```python
from build123d import *

# Parameters (mm, degrees)
F0_W     = 37
F0_H     = 69
F1_DEPTH = 5


with BuildPart() as f1:
    # F0 (on Top) → F1 (new body)
    with BuildSketch(Plane.XY):
        Polygon((109.757393, -47.013952), (-190.469548, -47.013952), (-187.938355, -69.176264), (-184.088363, -77.644812), (-178.970914, -85.570573), (-173.10958, -92.22553), (-166.061834, -97.942505), (-158.033386, -102.625757), (-150.505585, -106.763709), (-142.395731, -109.967075), (-134.17314, -111.816847), (-125.182951, -113.624161), (-117.335529, -114.393513), (-110.297666, -113.927758), (-97.994511, -110.570822), (-84.98137, -104.478377), (-74.645462, -98.277857), (-61.347514, -92.467954), (-54.509754, -89.918709), (-46.818863, -88.209901), (-39.777415, -88.209901), (-33.070793, -88.209901), (-25.985741, -90.074082), (-18.618021, -92.997303), (-10.935776, -97.133205), (-1.40856, -104.7078), (7.10493, -112.998784), (15.743346, -121.422512), (21.768701, -126.512042), (30.47871, -133.017234), (39.396258, -138.681565), (50.354269, -144.791737), (60.591184, -149.491585), (74.199441, -154.41068), (89.423326, -158.059629), (98.85233, -159.107134), (106.677154, -159.976425), (116.486558, -159.976425), (126.872966, -159.103989), (140.423232, -157.318581), (153.42437, -154.017258), (167.162878, -148.336862), (175.342116, -143.532352), (185.6123, -136.302521), (195.518968, -128.048335), (204.653845, -117.358152), (213.371967, -105.595887), (220.455531, -93.514166), (225.775129, -81.625274), (230.597933, -67.78821), (233.441157, -55.785481), (235.624263, -44.975688), (236.896344, -20.704121), (236.86714, -9.510057), (236.86714, 1.11357), (235.906968, 22.984027), (233.25353, 44.31771), (229.252552, 63.059144), (223.510394, 79.554792), (216.840677, 92.894226), (207.739533, 107.33053), (197.024369, 120.1263), (184.641449, 131.468644), (171.094149, 140.879356), (153.60487, 149.05483), (132.97725, 154.472187), (114.898965, 156.457659), (99.067456, 156.457659), (84.663291, 154.488749), (66.679821, 149.783781), (53.734493, 144.398522), (42.264603, 138.037948), (27.751352, 128.291809), (16.359527, 119.536983), (4.246612, 108.496011), (-5.338126, 100.151649), (-13.215689, 95.496727), (-20.495536, 92.632523), (-29.407222, 90.433524), (-36.891697, 89.410468), (-42.068154, 89.410468), (-50.267792, 90.919179), (-59.070143, 93.618111), (-68.10425, 98.191586), (-78.777898, 104.228198), (-85.258181, 107.363312), (-92.926764, 110.724328), (-100.445934, 113.46735), (-107.684615, 114.975152), (-115.831575, 115.993351), (-123.636163, 115.993351), (-129.309204, 115.993351), (-133.603284, 114.941916), (-137.040821, 113.433007), (-138.448742, 112.306855), (-139.140668, 111.03855), (-139.344401, 110.549672), (-138.28696, 108.284083), (-136.043459, 105.957887), (-131.906646, 102.131959), (-126.94568, 97.960933), (-121.69705, 91.98096), (-117.6631, 84.796643), (-115.553754, 76.732782), (-114.52125, 64.899556), (-115.629325, 56.405594), (-116.508421, 53.80871), (109.757393, 52.986048), align=None)
        Polygon((241.896685, -20.828539), (241.86714, -9.503535), (241.86714, 1.223274), (240.893394, 23.402912), (238.188565, 45.149782), (234.077219, 64.408205), (228.126581, 81.502758), (221.202205, 95.35151), (211.789387, 110.282193), (200.645468, 123.589971), (187.770458, 135.383053), (173.597124, 145.228644), (155.312446, 153.775932), (133.890159, 159.40199), (115.172707, 161.457659), (98.727311, 161.457659), (83.688435, 159.40199), (65.079178, 154.533299), (51.555006, 148.90724), (39.653731, 142.307444), (24.831248, 132.353646), (13.146367, 123.3736), (0.920512, 112.229684), (-8.275919, 104.223377), (-15.416681, 100.003837), (-22.016478, 97.407195), (-30.347364, 95.35151), (-37.231842, 94.410468), (-41.61199, 94.410468), (-49.078566, 95.784297), (-57.194419, 98.27274), (-65.74312, 102.60048), (-76.456041, 108.659303), (-83.165131, 111.905112), (-91.064569, 115.367308), (-99.0722, 118.288523), (-106.86343, 119.91142), (-115.520338, 120.993351), (-123.636163, 120.993351), (-129.912436, 120.993351), (-135.214792, 119.695033), (-139.651454, 117.747557), (-142.356729, 115.583694), (-143.655285, 113.20343), (-144.737394, 110.606795), (-143.979894, 108.659303), (-142.464952, 105.413509), (-139.543231, 102.384094), (-135.214792, 98.38094), (-130.45349, 94.377787), (-125.800382, 89.076315), (-122.337637, 82.909292), (-120.498056, 75.876723), (-119.549613, 65.006897), (-120.5235, 57.541555), (-121.780652, 53.827879), (-116.508421, 53.80871), (-115.629325, 56.405594), (-114.52125, 64.899556), (-115.553754, 76.732782), (-117.6631, 84.796643), (-121.69705, 91.98096), (-126.94568, 97.960933), (-131.906646, 102.131959), (-136.043459, 105.957887), (-138.28696, 108.284083), (-139.344401, 110.549672), (-139.140668, 111.03855), (-138.448742, 112.306855), (-137.040821, 113.433007), (-133.603284, 114.941916), (-129.309204, 115.993351), (-123.636163, 115.993351), (-115.831575, 115.993351), (-107.684615, 114.975152), (-100.445934, 113.46735), (-92.926764, 110.724328), (-85.258181, 107.363312), (-78.777898, 104.228198), (-68.10425, 98.191586), (-59.070143, 93.618111), (-50.267792, 90.919179), (-42.068154, 89.410468), (-36.891697, 89.410468), (-29.407222, 90.433524), (-20.495536, 92.632523), (-13.215689, 95.496727), (-5.338126, 100.151649), (4.246612, 108.496011), (16.359527, 119.536983), (27.751352, 128.291809), (42.264603, 138.037948), (53.734493, 144.398522), (66.679821, 149.783781), (84.663291, 154.488749), (99.067456, 156.457659), (114.898965, 156.457659), (132.97725, 154.472187), (153.60487, 149.05483), (171.094149, 140.879356), (184.641449, 131.468644), (197.024369, 120.1263), (207.739533, 107.33053), (216.840677, 92.894226), (223.510394, 79.554792), (229.252552, 63.059144), (233.25353, 44.31771), (235.906968, 22.984027), (236.86714, 1.11357), (236.86714, -9.510057), (236.896344, -20.704121), (235.624263, -44.975688), (233.441157, -55.785481), (230.597933, -67.78821), (225.775129, -81.625274), (220.455531, -93.514166), (213.371967, -105.595887), (204.653845, -117.358152), (195.518968, -128.048335), (185.6123, -136.302521), (175.342116, -143.532352), (167.162878, -148.336862), (153.42437, -154.017258), (140.423232, -157.318581), (126.872966, -159.103989), (116.486558, -159.976425), (106.677154, -159.976425), (98.85233, -159.107134), (89.423326, -158.059629), (74.199441, -154.41068), (60.591184, -149.491585), (50.354269, -144.791737), (39.396258, -138.681565), (30.47871, -133.017234), (21.768701, -126.512042), (15.743346, -121.422512), (7.10493, -112.998784), (-1.40856, -104.7078), (-10.935776, -97.133205), (-18.618021, -92.997303), (-25.985741, -90.074082), (-33.070793, -88.209901), (-39.777415, -88.209901), (-46.818863, -88.209901), (-54.509754, -89.918709), (-61.347514, -92.467954), (-74.645462, -98.277857), (-84.98137, -104.478377), (-97.994511, -110.570822), (-110.297666, -113.927758), (-117.335529, -114.393513), (-125.182951, -113.624161), (-134.17314, -111.816847), (-142.395731, -109.967075), (-150.505585, -106.763709), (-158.033386, -102.625757), (-166.061834, -97.942505), (-173.10958, -92.22553), (-178.970914, -85.570573), (-184.088363, -77.644812), (-187.938355, -69.176264), (-190.469548, -47.013952), (-195.502055, -47.013952), (-192.816544, -70.52742), (-188.488075, -80.048439), (-182.969332, -88.595711), (-176.584836, -95.844667), (-168.913197, -102.06773), (-160.497736, -106.976739), (-152.636803, -111.29781), (-143.871701, -114.759998), (-135.214792, -116.707474), (-125.921469, -118.575728), (-117.414903, -119.409702), (-109.466198, -118.883669), (-96.263724, -115.281352), (-82.629097, -108.897942), (-72.349024, -102.730918), (-59.471869, -97.10486), (-53.087402, -94.724611), (-46.270089, -93.2099), (-39.777415, -93.2099), (-33.717573, -93.2099), (-27.549523, -94.832804), (-20.732225, -97.53764), (-13.698481, -101.324407), (-4.716933, -108.46517), (3.615337, -116.57967), (12.380454, -125.12695), (18.656712, -130.428414), (27.638252, -137.136404), (36.836223, -142.978855), (48.090199, -149.254057), (58.694911, -154.122764), (72.762384, -159.207856), (88.561238, -162.994616), (98.300256, -164.076562), (106.400271, -164.976425), (116.696184, -164.976425), (127.409104, -164.076562), (141.368369, -162.237264), (155.002991, -158.775083), (169.3951, -152.824446), (178.052005, -147.739353), (188.656718, -140.274027), (199.045011, -131.618553), (208.567606, -120.474638), (217.549146, -108.356976), (224.907514, -95.80655), (230.426294, -83.472502), (235.404011, -69.190978), (238.325717, -56.856934), (240.598152, -45.604822), align=None)
        Polygon((-116.508421, 53.80871), (-121.780652, 53.827879), (-122.904166, 50.508979), (-127.016189, 43.6928), (-132.751377, 38.499518), (-140.001537, 33.739009), (-147.929535, 31.704532), (-134.216449, 31.556042), (-129.682809, 34.532863), (-123.114868, 40.480213), (-118.342329, 48.391277), (-117.044656, 52.224651), align=None)
        Polygon((-196.325026, -31.183951), (-195.502055, -47.013952), (-190.469548, -47.013952), (109.757393, -47.013952), (109.757393, 52.986048), (-116.508421, 53.80871), (-117.044656, 52.224651), (-118.342329, 48.391277), (-123.114868, 40.480213), (-129.682809, 34.532863), (-134.216449, 31.556042), (-113.145601, 31.327879), (-113.742607, -23.805663), (-196.325026, -23.068249), align=None)
        with Locations((-86.742607, 3.827879)):
            Rectangle(F0_W, F0_H, mode=Mode.SUBTRACT)
        with Locations((16.257393, 3.827879)):
            Rectangle(F0_W, F0_H, mode=Mode.SUBTRACT)
        Polygon((-168.913197, 31.931751), (-196.325026, -23.068249), (-113.742607, -23.805663), (-113.145601, 31.327879), (-134.216449, 31.556042), (-147.929535, 31.704532), align=None)
        with Locations((-86.742607, 3.827879)):
            Rectangle(F0_W, F0_H)
        with Locations((16.257393, 3.827879)):
            Rectangle(F0_W, F0_H)
    extrude(amount=F1_DEPTH)


solid = f1.part
```
Geometry check sheet. Reference: the model listing, model coordinates, mm. Round coordinates to 2 decimals unless told otherwise and drop trailing zeros. Loops run counter-clockwise (first coordinate to the right, second up) from the corner with the lowest first, then second, coordinate; pieces in that order, holes last. Notation, with made-up numbers: (-10.5, 73.5) -> (6.5, 73.5) arc R14 cw to (6.5, 81.5) -> close; hole circle Ø11 at (41.5, -28). An arc over 180 degrees is marked (long way). Use a Markdown table: item, result.
(1) Scan lines: probe 1 along Y at (x, z) = (189.5, 2.95); probe 2 along X at (y, z) = (103, 2.25); probe 3 along Y at (x, z) = (-108, 0.3). Record each from-to range of solid material in increasing order.
Calculated:
| item | result |
|---|---|
| probe 1 | -139.57 to 133.8 |
| probe 2 | -140.14 to -66.45, -10.35 to 216.38 |
| probe 3 | -118.48 to 120.05 |
(2) Mould release check, pull along X, two halves, no side actions. Record for faces 1 (the flat face through (7.12, 117.88, 2.46)), 2 (the flat face through (68, 1, 0)), 3 (the flat face through (32.346, 137.4, 2.465)), 4 (the flat face through (216.562, 102.712, 2.465)): released by +X, released by -X, zero draft, split by the parting line, or undercut.
Calculated:
| item | result |
|---|---|
| face 1 | undercut |
| face 2 | zero draft |
| face 3 | released by -X |
| face 4 | released by +X |
(3) Sectioned sample at A-A (y = -75). Enter the section's corners in (x, z), then the cut area to 3 significant figures.
Calculated:
| item | result |
|---|---|
| outline | (-190.78, 0) -> (233.38, 0) -> (233.38, 5) -> (-190.78, 5) -> close |
| area | 2,120 mm² |
(4) Go/stop test with flat-tipped pins: P1, Ø1, axis at x = -55, z = 4.5, coming from the +Y side; P2, Ø2, axis at x = -131.5, z = 3.5, coming from the +Y side; P3, Ø2, axis at y = -82, z = 2.5, coming from the +X side. Record where each tip stops, or that it passes through.
Calculated:
| item | result |
|---|---|
| P1 | y = 97.75 |
| P2 | y = 120.85 |
| P3 | x = 231.29 |
